Input: part model. Units: mm. Frame: model coordinates. A direction names the side the tool comes from. Coordinates: 2 decimals unless noted, no trailing zeros. Write each loop counter-clockwise with the first axis right and the second up, starting at its lowest first coordinate (ties: lowest second). Pieces come first, ordered by that corner, then holes. Notation, with made-up numbers: M 78.5,15 L 92.5,15 A22 ccw 92.5,48 Z; hole C 15,47 d11. An arc over 180 degrees is marked long. Answer as a JSON object with one key per item and string values. Group by question number.
from build123d import *

# Parameters (mm, degrees)
SKETCH_1_W          = 28
SKETCH_1_H          = 28
SKETCH_1_W_2        = 20.5
SKETCH_1_H_2        = 20.5
EXTRUDE_1_DEPTH     = 50
SKETCH_2_W          = 28
SKETCH_2_H          = 28
EXTRUDE_2_DEPTH     = 10
SKETCH_7_W          = 28
SKETCH_7_H          = 28
EXTRUDE_4_DEPTH     = 48
SKETCH_8_W          = 20
SKETCH_8_H          = 28
CUT_EXTRUDE_4_DEPTH = 20
FILLET_4_R          = 12
FILLET_6_R          = 2
SKETCH_9_R          = 2
CUT_EXTRUDE_5_DEPTH = 86.134031464
CUT_EXTRUDE_START   = -26.5
CUT_EXTRUDE_6_DEPTH = 59.634031464
SKETCH_12_R         = 2
CUT_EXTRUDE_7_DEPTH = 67.633324996


with BuildPart() as part:
    # 草图1 → 凸台-拉伸1 (new body)
    with BuildSketch(Plane.XY):
        Rectangle(SKETCH_1_W, SKETCH_1_H)
        Rectangle(SKETCH_1_W_2, SKETCH_1_H_2, mode=Mode.SUBTRACT)
    extrude(amount=EXTRUDE_1_DEPTH)

    # 草图2 → 凸台-拉伸2 (add)
    with BuildSketch(Plane(origin=(0, 0, 0), x_dir=(-1, 0, 0), z_dir=(0, 0, -1))):
        Rectangle(SKETCH_2_W, SKETCH_2_H)
    extrude(amount=-EXTRUDE_2_DEPTH)

    # 草图7 → 凸台-拉伸4 (add)
    with BuildSketch(Plane(origin=(14, 0, 0), x_dir=(0, 0, -1), z_dir=(1, 0, 0))):
        with Locations((12.784134516, 0)):
            Rectangle(SKETCH_7_W, SKETCH_7_H)
    extrude(amount=-EXTRUDE_4_DEPTH)

    # 草图8 → 切除-拉伸4 (cut)
    with BuildSketch(Plane.ZY.offset(34)):
        with Locations((-12.784134516, 0)):
            Rectangle(SKETCH_8_W, SKETCH_8_H)
    extrude(amount=-CUT_EXTRUDE_4_DEPTH, mode=Mode.SUBTRACT)

    # 圆角4
    fillet_4_edges = [part.edges().sort_by_distance(p)[0] for p in [
        (-14, 0, 1.215865484),
        (14, 0, -26.784134516),
    ]]
    fillet(fillet_4_edges, radius=FILLET_4_R)

    # 圆角6
    fillet_6_edges = [part.edges().sort_by_distance(p)[0] for p in [
        (-34, 0, 1.215865484),
        (-30, -14, 1.215865484),
        (-30, 14, 1.215865484),
        (-34, 0, -26.784134516),
        (-16, 14, -26.784134516),
        (-16, -14, -26.784134516),
        (14, -14, 17.607932742),
        (-14, -14, 31.607932742),
        (-14, 14, 31.607932742),
        (14, 14, 17.607932742),
        (10.485281374, 14, -23.26941589),
        (10.485281374, -14, -23.26941589),
        (-17.514718626, -14, 4.73058411),
        (-17.514718626, 14, 4.73058411),
    ]]
    fillet(fillet_6_edges, radius=FILLET_6_R)

    # 草图9 → 切除-拉伸5 (cut, through all)
    with BuildSketch(Plane(origin=(0, 0, -26.784134516), x_dir=(-1, 0, 0), z_dir=(0, 0, -1))):
        with Locations((24, 7.5)):
            Circle(SKETCH_9_R)
        with Locations((24, -7.5)):
            Circle(SKETCH_9_R)
    extrude(amount=-CUT_EXTRUDE_5_DEPTH, mode=Mode.SUBTRACT)

    # 草图10 → 切除-拉伸6 (cut, through all)
    with BuildSketch(Plane(origin=(0, 0, -26.784134516), x_dir=(-1, 0, 0), z_dir=(0, 0, -1)).offset(CUT_EXTRUDE_START)):
        Polygon((19.669872981, 7.5), (21.834936491, 3.75), (26.165063509, 3.75), (28.330127019, 7.5), (26.165063509, 11.25), (21.834936491, 11.25), align=None)
        Polygon((19.669872981, -7.5), (21.834936491, -11.25), (26.165063509, -11.25), (28.330127019, -7.5), (26.165063509, -3.75), (21.834936491, -3.75), align=None)
    extrude(amount=-CUT_EXTRUDE_6_DEPTH, mode=Mode.SUBTRACT)

    # 草图12 → 切除-拉伸7 (cut, through all)
    with BuildSketch(Plane(origin=(0, 14, 0), x_dir=(1, 0, 0), z_dir=(0, 1, 0))):
        with Locations(Location((0, -40, 0), (0, 0, 270))):
            Circle(SKETCH_12_R)
        with Locations(Location((0, -20, 0), (0, 0, 270))):
            Circle(SKETCH_12_R)
    extrude(amount=-CUT_EXTRUDE_7_DEPTH, mode=Mode.SUBTRACT)


solid = part.part
Q1. Draft query along Y for faces 4 (the cylindrical face through (0, 12, 38)), 5 (the cylindrical face through (13.4, 13.43, 17.15)), 6 (the flat face through (-24, 11.25, 1)). Return one class per face: released by +Y, released by -Y, zero draft, split by the parting line, or undercut.
Q2. Section D-D, the plane y = -1.5. Return the cut outline in (x, z).
Q3. Section C-C, the plane z = 37. Return the cut outline in (x, y), and give its area (3 significant figures).
Q4. Section B-B, the plane z = 20. Return the cut outline in (x, y), and give its area (3 significant figures).
Q5. Pin query (flat end, axial travel): pin 1 Ø6 at (x, y) = (-20, -4.5) entering from +Z; pin 2 Ø0.7 at (x, z) = (-23.5, 1) entering from -Y; pin 3 Ø5 at (y, z) = (-10, 14) entering from -X. Return the tip coordinate at first contact, or that it passes through.
Q6. Line query: line 1 (Y direction, x = -24, z = -1); line 2 (X direction, y = 3.5, z = 29.5). Output: solid intervals per line, ascending. Write a range as from..to.
Q7. Section A-A, the plane x = -5. Return the cut outline in (y, z).
Q8. Access query for faces 1 (the flat face through (0, -10.25, 30)), 2 (the flat face through (-30, 0, 1.216)), 3 (the flat face through (-14, 0, -13)). Directions: +Z, -Z, +X, -X, +Y, -Y. A direction counts if a zero-diameter tool reaches every point of the face in a straight line with its end or side. Return the directions, or none.
Filled in:
{
 "1": {"face 4": "zero draft", "face 5": "released by +Y", "face 6": "undercut"},
 "2": {"outline": "M -34,-24.78 A2 ccw -32,-26.78 L 2,-26.78 A12 ccw 14,-14.78 L 14,50 L 10.25,50 L 10.25,10 L -10.25,10 L -10.25,50 L -14,50 L -14,13.22 A12 cw -26,1.22 L -32,1.22 A2 ccw -34,-0.78 L -34,-2.78 L -14,-2.78 L -14,-22.78 L -34,-22.78 Z"},
 "3": {"outline": "M -14,-12 A2 ccw -12,-14 L 12,-14 A2 ccw 14,-12 L 14,12 A2 ccw 12,14 L -12,14 A2 ccw -14,12 Z; hole M -10.25,-10.25 L 10.25,-10.25 L 10.25,10.25 L -10.25,10.25 Z", "area": "360 mm^2"},
 "4": {"outline": "M -14,-12 A2 ccw -12,-14 L -2,-14 L -2,-10.25 L -10.25,-10.25 L -10.25,10.25 L -2,10.25 L -2,14 L -12,14 A2 ccw -14,12 Z; M 2,-14 L 12,-14 A2 ccw 14,-12 L 14,12 A2 ccw 12,14 L 2,14 L 2,10.25 L 10.25,10.25 L 10.25,-10.25 L 2,-10.25 Z", "area": "330 mm^2"},
 "5": {"pin 1": "z = 5.28", "pin 2": "y = -13.61", "pin 3": "x = -14.12"},
 "6": {"line 1": "-14..-9.5, -5.5..5.5, 9.5..14", "line 2": "-14..-10.25, 10.25..14"},
 "7": {"outline": "M -14,-24.78 A2 ccw -12,-26.78 L 12,-26.78 A2 ccw 14,-24.78 L 14,50 L 10.25,50 L 10.25,10 L -10.25,10 L -10.25,50 L -14,50 Z"},
 "8": {"face 1": "+Z", "face 2": "+Z, -X, +Y, -Y", "face 3": "-X, +Y, -Y"}
}
